For this review, use the dimensioned drawing (mm, ordinates from the lowest corner) and the shaded views. Round coordinates to 2 decimals unless told otherwise and drop trailing zeros. Order: outer loops, then holes, each group sorted by start corner. A loop starts at its lowest first (then second) coordinate and runs counter-clockwise, first axis right, second up. Notation, with made-up numbers: (19.5, 57.5) - (35.5, 57.5) arc R3 cw to (35.5, 62.5) - close; hole circle Ø4 at (46.5, -34.5). An arc over 180 degrees is marked (long way). Write item = value, one per line.
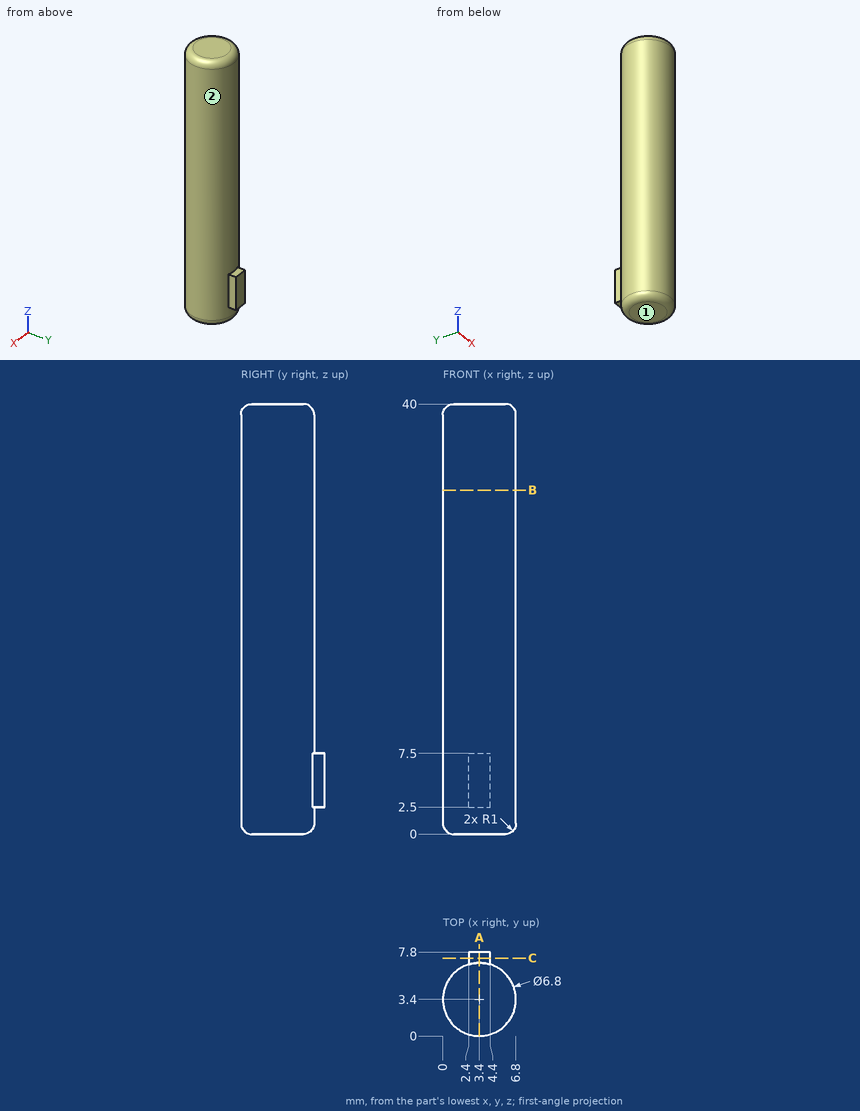
1) The part is to be moulded in two halves that separate along X. For the marked faces 1 and 2, say which applies: released by +X, released by -X, zero draft, split by the parting line, or undercut.
Findings:
face_1 = zero draft
face_2 = split by the parting line
2) We need section C-C on y = 7.25. Write out the cut boundary in (x, z).
Findings:
outline = (2.4, 2.5) - (4.4, 2.5) - (4.4, 7.5) - (2.4, 7.5) - close
3) Clearance check with flat-ended pins moving along their axes: pin 1 Ø0.6 at (x, y) = (3, 7.5) entering from -Z; pin 2 Ø1 at (x, z) = (1, 34) entering from -Y; pin 3 Ø1.3 at (y, z) = (7, 6) entering from +X. State where each tip first meets the part, or that it passes through.
Findings:
pin_1 = 2.5
pin_2 = 0.58
pin_3 = 5.09
4) To check wall thickness, follow L1, parallel to Y at x = 1, z = 4.5; L2, parallel to Y at x = 3.5, z = 24. State the ranges of each line that lie inside material, in increasing order. Write a range as from..to.
Findings:
L1 = 0.99..5.81
L2 = 0..6.8
5) We need section A-A on x = 3.4. Write out the cut boundary in (y, z).
Findings:
outline = (0, 1) arc R1 ccw to (1, 0) - (5.8, 0) arc R1 ccw to (6.8, 1) - (6.8, 2.5) - (7.8, 2.5) - (7.8, 7.5) - (6.8, 7.5) - (6.8, 39) arc R1 ccw to (5.8, 40) - (1, 40) arc R1 ccw to (0, 39) - close
6) We need section B-B on z = 32. Write out the cut boundary in (x, y).
Findings:
outline = circle Ø6.8 at (3.4, 3.4)
